from build123d import *

# Parameters (mm, degrees)
ESBO_O1_R                = 44.5
ESBO_O1_R_2              = 36.4
RESSALTO_EXTRUS_O1_DEPTH = 275
CHANFRO1_SIZE            = 1
ESBO_O5_R                = 1
CORTE_EXTRUS_O3_DEPTH    = 293.448713452
ESBO_O13_R               = 1
CORTE_EXTRUS_O4_DEPTH    = 293.448713592


with BuildPart() as part:
    # Esboço1 → Ressalto-extrusão1 (new body)
    with BuildSketch(Plane(origin=(0, 0, 0), x_dir=(1, 0, 0), z_dir=(0, 1, 0))):
        with Locations(Location((0, 0, 0), (0, 0, 270))):
            Circle(ESBO_O1_R)
        with Locations(Location((0, 0, 0), (0, 0, 270))):
            Circle(ESBO_O1_R_2, mode=Mode.SUBTRACT)
    extrude(amount=RESSALTO_EXTRUS_O1_DEPTH)

    # Chanfro1
    chanfro1_edges = [part.edges().sort_by_distance(p)[0] for p in [
        (0, 0, -36.4),
        (0, 275, -36.4),
    ]]
    chamfer(chanfro1_edges, length=CHANFRO1_SIZE)

    # Esboço5 → Corte-extrusão3 (cut, through all)
    with BuildSketch(Plane.XY.offset(44.5)):
        with Locations((0, 269.75)):
            Circle(ESBO_O5_R)
        with Locations((0, 5.25)):
            Circle(ESBO_O5_R)
    extrude(amount=-CORTE_EXTRUS_O3_DEPTH, mode=Mode.SUBTRACT)

    # Esboço13 → Corte-extrusão4 (cut, through all)
    with BuildSketch(Plane.ZY.offset(44.5)):
        with Locations((0, 5.25)):
            Circle(ESBO_O13_R)
        with Locations((0, 269.75)):
            Circle(ESBO_O13_R)
    extrude(amount=-CORTE_EXTRUS_O4_DEPTH, mode=Mode.SUBTRACT)


solid = part.part
Source: CAD feature listing. Evaluate the final solid. Frame: model axes, mm. Round coordinates to 2 decimals unless told otherwise and drop trailing zeros. Loops run counter-clockwise (first coordinate to the right, second up) from the corner with the lowest first, then second, coordinate; pieces in that order, holes last. Notation, with made-up numbers: (25.25, 59.5) - (45.25, 59.5) arc R18 ccw to (45.25, 87.5) - close; hole circle Ø1 at (-0.5, -6.75). An arc over 180 degrees is marked (long way). Write item = value, one per line. Start each with the question number.
(1) Section query A-A, the plane y = 38. Output: boundary loops of the cut face in (x, z), plus the area to 3 significant figures.
(2) Ray query, line 1 along Y through (x, z) = (0, 38.25); line 2 along X through (y, z) = (159, 0); line 3 along Z through (x, y) = (19, 34). Return the intervals inside material, ascending. Write a range as from..to.
(3) Pin query (flat end, axial travel): pin 1 (3 mm diameter, centred on y = 246.5, z = -23.5, fed in from -X); pin 2 (2 mm diameter, centred on x = 34.5, y = 34, fed in from +Z); pin 3 (8 mm diameter, centred on x = 27, y = 159, fed in from +Z). Return the tip coordinate at first contact, or that it passes through.
(4) Pull-direction query (Z, two-part tool) for faces 1 (the face through (36.5, 0, -10.1)), 2 (the face through (30.075, 135.575, -32.798)), 3 (the face through (-22, 136, -29)); classes: +Z half, -Z half, draft (parallel to the pull), parting line (faces both ways), or undercut.
Conclusion:
q1.outline = circle Ø89 at (0, 0); hole circle Ø72.8 at (0, 0)
q1.area = 2,060 mm2
q2.line_1 = 0..4.25, 6.25..268.75, 270.75..275
q2.line_2 = -44.5..-36.4, 36.4..44.5
q2.line_3 = -40.24..-31.05, 31.05..40.24
q3.pin_1 = -38.68
q3.pin_2 = 29.29
q3.pin_3 = 38.1
q4.face_1 = draft
q4.face_2 = parting line
q4.face_3 = undercut
